```python
from build123d import *

# Parameters (mm, degrees)
F0_W      = 30
F0_H      = 18
F1_DEPTH  = 30
F3_W      = 20
F3_H      = 20
F5_DEPTH  = 10
F4_R      = 3.5
F6_DEPTH  = 46
F9_R      = 0.5
F7_R      = 3.5
F11_R     = 1.3
F12_DEPTH = 8


with BuildPart() as f1:
    # F0 (on Top) → F1 (new body)
    with BuildSketch(Plane.XY):
        Rectangle(F0_W, F0_H)
    extrude(amount=F1_DEPTH)



with BuildPart() as f5:
    # F3 (on offset) → F5 (new body)
    with BuildSketch(Plane.XY.offset(-6)):
        with Locations((0, -1)):
            Rectangle(F3_W, F3_H)
    extrude(amount=-F5_DEPTH)


with BuildPart() as f1_1:
    add(f1.part)

    add(f5.part)  # F6 merges F5
    # F4 (on face) → F6 (join, through all)
    with BuildSketch(Plane.XY.offset(30)):
        with Locations((0, 3)):
            Circle(F4_R)
    extrude(amount=-F6_DEPTH)

    # F9 (on offset) → F10 section 0
    with BuildSketch(Plane.XY.offset(-21.5)):
        with Locations((0, 3)):
            Circle(F9_R)
    # F7 (on face) → F10 section 1
    with BuildSketch(Plane(origin=(0, 0, -16), x_dir=(1, 0, 0), z_dir=(0, 0, -1))):
        with Locations((0, -3)):
            Circle(F7_R)
    loft()

    # F11 (on face) → F12 (cut)
    with BuildSketch(Plane.XY.offset(30)):
        with Locations((-8.5, 6)):
            Circle(F11_R)
        with Locations((8.5, 6)):
            Circle(F11_R)
        with Locations((8.5, -6)):
            Circle(F11_R)
        with Locations((-8.5, -6)):
            Circle(F11_R)
    extrude(amount=-F12_DEPTH, mode=Mode.SUBTRACT)


solid = f1_1.part
```
Input: part model. Units: mm. Frame: model coordinates. A direction names the side the tool comes from. Round coordinates to 2 decimals unless told otherwise and drop trailing zeros. Loops run counter-clockwise (first coordinate to the right, second up) from the corner with the lowest first, then second, coordinate; pieces in that order, holes last. Notation, with made-up numbers: M 7,17 L 15,17 A17 cw 15,31 Z; hole C 28.5,-15.5 d4. An arc over 180 degrees is marked long. Answer in a Markdown table with one row per item. Add a question column.
1. Contact query for flat-ended pins moving along their axis: pin 1 (1.6 mm diameter, centred on x = 8.5, y = 6, fed in from -Z); pin 2 (3 mm diameter, centred on y = -1.5, z = -11.5, fed in from -X); pin 3 (8 mm diameter, centred on y = 1, z = -10, fed in from +X). Output: stop coordinate, or through.
2. Mould query, pull axis Z, two halves, no side actions, for faces 4 (the face through (0.907, 4.423, -19.323)), 5 (the face through (0, -2, 0)), 6 (the face through (10, -1, -11)). Classes: released by +Z, released by -Z, zero draft, split by the parting line, or undercut.
3. Section C-C (z = 25.5). Output: boundary loops of the cut face in (x, y).
4. Section A-A (x = -8.5). Output: boundary loops of the cut face in (y, z).
5. Ray query, probe 1 along Y at (x, z) = (-8.5, 27.75); probe 2 along Z at (x, y) = (-4, -1); probe 3 along Z at (x, y) = (-9.5, -6.25). Return the intervals inside material, ascending.
6. Set-up query: faces 1 (the face through (-7.9, 4.847, 26.056)), 2 (the face through (0, -9, 15)), 3 (the face through (-10, -1, -11)). Return all of +Z, -Z, +X, -X, +Y, -Y with unobstructed straight access to the full face (end or side cutting, diameter ignored); none if empty.
7. Section D-D (x = 11.25). Output: boundary loops of the cut face in (y, z).
8. Section B-B (y = -6). Output: boundary loops of the cut face in (x, z), and give its area (3 significant figures).
Values follow:
| question | item | result |
|---|---|---|
| 1 | pin 1 | z = -16 |
| 1 | pin 2 | x = -10 |
| 1 | pin 3 | x = 10 |
| 2 | face 4 | released by -Z |
| 2 | face 5 | undercut |
| 2 | face 6 | zero draft |
| 3 | outline | M -15,-9 L 15,-9 L 15,9 L -15,9 Z; hole C -8.5,-6 d2.6; hole C -8.5,6 d2.6; hole C 8.5,-6 d2.6; hole C 8.5,6 d2.6 |
| 4 | outline | M -11,-16 L 9,-16 L 9,-6 L -11,-6 Z; M -9,0 L 9,0 L 9,30 L 7.3,30 L 7.3,22 L 4.7,22 L 4.7,30 L -4.7,30 L -4.7,22 L -7.3,22 L -7.3,30 L -9,30 Z |
| 5 | probe 1 | -9 to -7.3, -4.7 to 4.7, 7.3 to 9 |
| 5 | probe 2 | -16 to -6, 0 to 30 |
| 5 | probe 3 | -16 to -6, 0 to 22 |
| 6 | face 1 | +Z |
| 6 | face 2 | +Z, +X, -X, -Y |
| 6 | face 3 | -Z, -X, +Y, -Y |
| 7 | outline | M -9,0 L 9,0 L 9,30 L -9,30 Z |
| 8 | outline | M -15,0 L 15,0 L 15,30 L 9.8,30 L 9.8,22 L 7.2,22 L 7.2,30 L -7.2,30 L -7.2,22 L -9.8,22 L -9.8,30 L -15,30 Z; M -10,-16 L 10,-16 L 10,-6 L -10,-6 Z |
| 8 | area | 1,060 mm^2 |
